```python
from build123d import *

# Parameters (mm, degrees)
F1_W     = 50.8
F1_H     = 50.8
F1_W_2   = 44.45
F1_H_2   = 44.45
F2_DEPTH = 304.8
F4_DEPTH = 50.801
F6_DEPTH = 127
F7_R     = 19.05
F8_DEPTH = 50.8


with BuildPart() as f2:
    # F1 (on face) → F2 (new body)
    with BuildSketch(Plane.XZ):
        Rectangle(F1_W, F1_H)
        Rectangle(F1_W_2, F1_H_2, mode=Mode.SUBTRACT)
    extrude(amount=F2_DEPTH)

    # F3 (on face) → F4 (cut, through all)
    with BuildSketch(Plane.YZ.offset(25.4)):
        Polygon((-283.757951, 25.4), (-304.8, 25.4), (-304.8, -25.4), align=None)
    extrude(amount=-F4_DEPTH, mode=Mode.SUBTRACT)

    # F5 (on face) → F6 (cut)
    with BuildSketch(Plane.YZ.offset(25.4)):
        Polygon((0, -25.4), (0, 25.4), (-21.042049, 25.4), align=None)
    extrude(amount=-F6_DEPTH, mode=Mode.SUBTRACT)

    # F7 (on face) → F8 (cut)
    with BuildSketch(Plane.XY.offset(25.4)):
        with Locations((0, -50.709249)):
            Circle(F7_R)
        with Locations((0, -101.885025)):
            Circle(F7_R)
        with Locations((0, -153.060801)):
            Circle(F7_R)
        with Locations((0, -204.236577)):
            Circle(F7_R)
        with Locations((0, -255.412352)):
            Circle(F7_R)
    extrude(amount=-F8_DEPTH, mode=Mode.SUBTRACT)


solid = f2.part
```
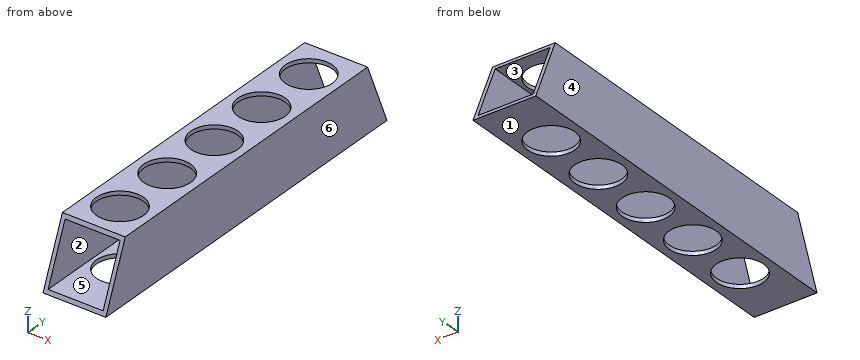
Work out the finished part from the listing and answer in its coordinate system (mm). Face numbers are marked on the shaded views. A direction names the side the tool comes from. Give positions to 0.01 mm unless a question says otherwise; leave off trailing zeros. Loops run counter-clockwise (first coordinate to the right, second up) from the corner with the lowest first, then second, coordinate; pieces in that order, holes last. Notation, with made-up numbers: (14, 69) - (23, 69) arc R20 ccw to (23, 98) - close; hole circle Ø1 at (37.25, -29.5). An arc over 180 degrees is marked (long way). Use CSV: the item, a comma, the result in double quotes. Start each with the question number.
(1) Find section A-A, the plane y = -280. Determine the outline of the cut face in (x, z) (3 decimals).
(2) Find the intervals of material crossed by L1, parallel to Z at x = -21, y = -103 (3 decimals); L2, parallel to Y at x = 0, z = 24.25, in increasing order.
(3) Find section C-C, the plane z = 17. Determine the outline of the cut face in (x, y) (3 decimals), plus the area to 3 significant figures.
(4) Each of these flat-tipped pins is pushed along its axis until it touches: pin 1 (23 mm diameter, centred on x = 0, y = -204.24, fed in from +Z); pin 2 (10 mm diameter, centred on x = 20, z = -14.5, fed in from +Y). Where does it stop, or does it pass through?
(5) Find section B-B, the plane y = -99. Determine the outline of the cut face in (x, z) (3 decimals).
(6) Find section D-D, the plane x = 0. Count the separate pieces of the cut face and the enclosed holes in it, plus the area to 3 significant figures.
(7) Determine the mould class of the marked faces 1, 2, 3 and 4 for opening direction X: released by +X, released by -X, zero draft, split by the parting line, or undercut.
(8) A tool of negligible diameter and unlimited length cuts with its end or side. For the marked faces 5 and 6, from which of +Z, -Z, +X, -X, +Y, -Y can it reach the whole face along a straight path? Write none if from no direction.
Results found:
1,outline,"(-25.4, -25.4) - (25.4, -25.4) - (25.4, 25.4) - (-25.4, 25.4) - close; hole (-22.225, -22.225) - (22.225, -22.225) - (22.225, 22.225) - (-22.225, 22.225) - close"
2,L1,"-25.4 to -22.225, 22.225 to 25.4"
2,L2,"-284.23 to -274.46, -236.36 to -223.29, -185.19 to -172.11, -134.01 to -120.94, -82.84 to -69.76, -31.66 to -20.57"
3,outline,"(-25.4, -287.237) - (-22.225, -287.237) - (-22.225, -17.563) - (-25.4, -17.563) - close; (22.225, -287.237) - (25.4, -287.237) - (25.4, -17.563) - (22.225, -17.563) - close"
3,area,"1,710 mm^2"
4,pin 1,"through"
4,pin 2,"y = -2.66"
5,outline,"(-25.4, -25.4) - (-18.83, -25.4) - (-18.83, -22.225) - (-22.225, -22.225) - (-22.225, 22.225) - (-18.83, 22.225) - (-18.83, 25.4) - (-25.4, 25.4) - close; (18.83, -25.4) - (25.4, -25.4) - (25.4, 25.4) - (18.83, 25.4) - (18.83, 22.225) - (22.225, 22.225) - (22.225, -22.225) - (18.83, -22.225) - close"
6,separate pieces,"12"
6,enclosed holes,"0"
6,area,"592 mm^2"
7,face 1,"zero draft"
7,face 2,"undercut"
7,face 3,"undercut"
7,face 4,"released by -X"
8,face 5,"+Y, -Y"
8,face 6,"+Z, -Z, +X, +Y, -Y"
